For this review, take the finished solid that the model builds, in its own axes (mm). Face numbers are marked on the shaded views. A direction names the side the tool comes from. Coordinates: 2 decimals unless noted, no trailing zeros. Write each loop counter-clockwise with the first axis right and the second up, starting at its lowest first coordinate (ties: lowest second). Pieces come first, ordered by that corner, then holes. Notation, with made-up numbers: (16.25, 30.5) - (55.25, 30.5) arc R17 ccw to (55.25, 60.5) - close; hole circle Ø5 at (1, 84.5). An arc over 180 degrees is marked (long way). Write each question's results on one line, items separated by ' | '.
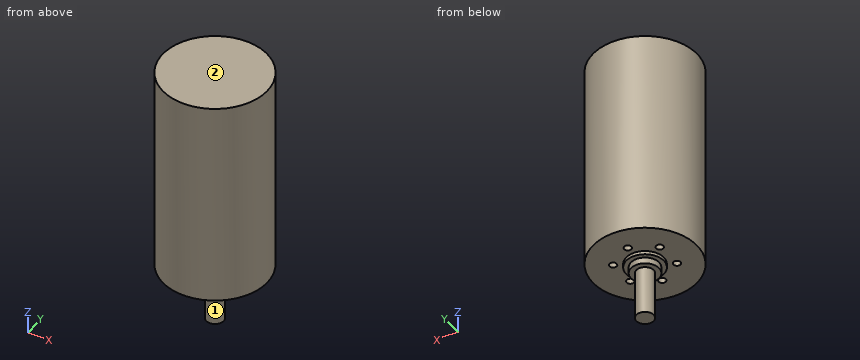
from build123d import *

# Parameters (mm, degrees)
SKETCH2_R          = 1.25
CUT_EXTRUDE1_DEPTH = 6.5


with BuildPart() as part:
    # Sketch1 → Revolve1 (revolve)
    with BuildSketch(Plane(origin=(0, 0, 0), x_dir=(0, 0, -1), z_dir=(1, 0, 0))):
        Polygon((0, 0), (0, 18), (71.3, 18), (71.3, 6.5), (72.5, 6.5), (72.5, 4.863636364), (74.65, 4.863636364), (74.65, 3), (91.3, 3), (91.3, 0), align=None)
    revolve(axis=Axis((0, 0, -91.3), (0, 0, 1)))

    # Sketch2 → Cut-Extrude1 (cut)
    with BuildSketch(Plane(origin=(0, 0, -71.3), x_dir=(-1, 0, 0), z_dir=(0, 0, -1))):
        with Locations((0, 9.5)):
            Circle(SKETCH2_R)
        with Locations((8.227241336, 4.75)):
            Circle(SKETCH2_R)
        with Locations((8.227241336, -4.75)):
            Circle(SKETCH2_R)
        with Locations((0, -9.5)):
            Circle(SKETCH2_R)
        with Locations((-8.227241336, -4.75)):
            Circle(SKETCH2_R)
        with Locations((-8.227241336, 4.75)):
            Circle(SKETCH2_R)
    extrude(amount=-CUT_EXTRUDE1_DEPTH, mode=Mode.SUBTRACT)


solid = part.part
Q1. Take a section at B-B on x = 0. State the section outline as (y, z) points, plus the area to 3 significant figures.
Results found:
outline: (-18, -71.3) - (-10.75, -71.3) - (-10.75, -64.8) - (-8.25, -64.8) - (-8.25, -71.3) - (-6.5, -71.3) - (-6.5, -72.5) - (-4.86, -72.5) - (-4.86, -74.65) - (-3, -74.65) - (-3, -91.3) - (3, -91.3) - (3, -74.65) - (4.86, -74.65) - (4.86, -72.5) - (6.5, -72.5) - (6.5, -71.3) - (8.25, -71.3) - (8.25, -64.8) - (10.75, -64.8) - (10.75, -71.3) - (18, -71.3) - (18, 0) - (-18, 0) - close | area: 2,670 mm2
Q2. Take a section at D-D on y = 9.5. State the section outline as (x, z) points.
Results found:
outline: (-15.29, -71.3) - (-1.25, -71.3) - (-1.25, -64.8) - (1.25, -64.8) - (1.25, -71.3) - (15.29, -71.3) - (15.29, 0) - (-15.29, 0) - close
Q3. Take a section at C-C on z = -82. State the section outline as (x, y) points.
Results found:
outline: circle Ø6 at (0, 0)
Q4. For the marked faces 1 and 2, list the 3-axis set-ups (+Z, -Z, +X, -X, +Y, -Y) from which the entire face can be reached by the end or side of a thin tool; tool diameter is ignored.
Results found:
face 1: -Z | face 2: +Z, +X, -X, +Y, -Y
Q5. For pin 1 (10 mm diameter, centred on y = -6, z = -57.5, fed in from -X); pin 2 (2 mm diameter, centred on x = -9, y = 5, fed in from -Z); pin 3 (1.2 mm diameter, centred on x = -8, y = -4.5, fed in from -Z), all flat-tipped, find the tip position at first contact; note any pin that passes through.
Results found:
pin 1: x = -17.97 | pin 2: z = -71.3 | pin 3: z = -64.8
Q6. Take a section at A-A on y = 0. State the section outline as (x, z) points.
Results found:
outline: (-18, -71.3) - (-6.5, -71.3) - (-6.5, -72.5) - (-4.86, -72.5) - (-4.86, -74.65) - (-3, -74.65) - (-3, -91.3) - (3, -91.3) - (3, -74.65) - (4.86, -74.65) - (4.86, -72.5) - (6.5, -72.5) - (6.5, -71.3) - (18, -71.3) - (18, 0) - (-18, 0) - close
Q7. Wall thickness on line 1 along Y through (x, z) = (0, -68); line 2 along X through (y, z) = (-4, -69); line 3 along X through (y, z) = (-9, -67): over which ranges is each line inside the solid? List them lowest first. Write a range as from..to.
Results found:
line 1: -18..-10.75, -8.25..8.25, 10.75..18 | line 2: -17.55..-9.23, -7.23..7.23, 9.23..17.55 | line 3: -15.59..-1.15, 1.15..15.59
